```python
from build123d import *

# Parameters (mm, degrees)
SKETCH1_W           = 88.9
SKETCH1_H           = 88.9
SKETCH1_W_2         = 76.2
SKETCH1_H_2         = 76.2
BOSS_EXTRUDE1_DEPTH = 50.8
SKETCH2_W           = 88.9
SKETCH2_H           = 88.9
BOSS_EXTRUDE2_DEPTH = 6.35
SKETCH3_W           = 12.7
SKETCH3_H           = 12.7
BOSS_EXTRUDE3_DEPTH = 6.35
SKETCH4_R           = 3.175
CUT_EXTRUDE1_DEPTH  = 58.15


with BuildPart() as part:
    # Sketch1 → Boss-Extrude1 (new body)
    with BuildSketch(Plane(origin=(0, 0, 0), x_dir=(1, 0, 0), z_dir=(0, 1, 0))):
        with Locations((38.1, 38.1)):
            Rectangle(SKETCH1_W, SKETCH1_H)
        with Locations((38.1, 38.1)):
            Rectangle(SKETCH1_W_2, SKETCH1_H_2, mode=Mode.SUBTRACT)
    extrude(amount=BOSS_EXTRUDE1_DEPTH)

    # Sketch2 → Boss-Extrude2 (add)
    with BuildSketch(Plane.XZ):
        with Locations((38.1, -38.1)):
            Rectangle(SKETCH2_W, SKETCH2_H)
    extrude(amount=BOSS_EXTRUDE2_DEPTH)

    # Sketch3 → Boss-Extrude3 (add)
    with BuildSketch(Plane(origin=(0, 50.8, 0), x_dir=(1, 0, 0), z_dir=(0, 1, 0))):
        with Locations((88.9, 38.1)):
            Rectangle(SKETCH3_W, SKETCH3_H)
        with Locations((-12.7, 38.1)):
            Rectangle(SKETCH3_W, SKETCH3_H)
    extrude(amount=-BOSS_EXTRUDE3_DEPTH)

    # Sketch4 → Cut-Extrude1 (cut, through all)
    with BuildSketch(Plane(origin=(0, 50.8, 0), x_dir=(1, 0, 0), z_dir=(0, 1, 0))):
        with Locations((88.9, 38.1)):
            Circle(SKETCH4_R)
        with Locations((-12.7, 38.1)):
            Circle(SKETCH4_R)
    extrude(amount=-CUT_EXTRUDE1_DEPTH, mode=Mode.SUBTRACT)


solid = part.part
```
Source: CAD feature listing. Evaluate the final solid. Frame: model axes, mm. A direction names the side the tool comes from. Round coordinates to 2 decimals unless told otherwise and drop trailing zeros. Loops run counter-clockwise (first coordinate to the right, second up) from the corner with the lowest first, then second, coordinate; pieces in that order, holes last. Notation, with made-up numbers: M -35.5,-36.5 L -18.5,-36.5 A19 cw -18.5,-9.5 Z; hole C 43,70 d7. An arc over 180 degrees is marked long. Put each result on its own line as item: value.
(1) Section D-D, the plane y = 46.5. Return loops of the section in (x, z) (3 decimals), and give its area (3 significant figures).
Solutions:
outline: M -19.05,-44.45 L -6.35,-44.45 L -6.35,-82.55 L 82.55,-82.55 L 82.55,-44.45 L 95.25,-44.45 L 95.25,-31.75 L 82.55,-31.75 L 82.55,6.35 L -6.35,6.35 L -6.35,-31.75 L -19.05,-31.75 Z; hole C -12.7,-38.1 d6.35; hole M 0,-76.2 L 76.2,-76.2 L 76.2,0 L 0,0 Z; hole C 88.9,-38.1 d6.35
area: 2,360 mm²
(2) First-contact query: pin 1 (3 mm diameter, centred on x = -10, y = 46, fed in from +Z); pin 2 (17 mm diameter, centred on y = 17.5, z = -26, fed in from -X); pin 3 (7 mm diameter, centred on x = -15.5, y = 47, fed in from -Z); pin 4 (4 mm diameter, centred on x = 88.9, z = -38.1, fed in from -Y). Flat tips, straight axial feed; report the tip coordinate or a pass-through.
Solutions:
pin 1: z = -31.75
pin 2: x = -6.35
pin 3: z = -44.45
pin 4: through
(3) Section B-B, the plane x = 88.9. Return loops of the section in (y, z) (3 decimals), and give its area (3 significant figures).
Solutions:
outline: M 44.45,-44.45 L 50.8,-44.45 L 50.8,-41.275 L 44.45,-41.275 Z; M 44.45,-34.925 L 50.8,-34.925 L 50.8,-31.75 L 44.45,-31.75 Z
area: 40.3 mm²
(4) Access query for faces 1 (the face through (-16, 44.45, -40)), 2 (the face through (38, 25, -76.2)), 3 (the face through (86, 44.45, -40)), 4 (the face through (89, 48, -44.45)). Directions: +Z, -Z, +X, -X, +Y, -Y. A direction counts if a zero-diameter tool reaches every point of the face in a straight line with its end or side. Return the directions, or none.
Solutions:
face 1: +Z, -Z, -X, -Y
face 2: +Y
face 3: +Z, -Z, +X, -Y
face 4: -Z, +X, +Y, -Y
(5) Section A-A, the plane z = -38.1. Return loops of the section in (x, y) (3 decimals), and give its area (3 significant figures).
Solutions:
outline: M -19.05,44.45 L -15.875,44.45 L -15.875,50.8 L -19.05,50.8 Z; M -9.525,44.45 L -6.35,44.45 L -6.35,-6.35 L 82.55,-6.35 L 82.55,44.45 L 85.725,44.45 L 85.725,50.8 L 76.2,50.8 L 76.2,0 L 0,0 L 0,50.8 L -9.525,50.8 Z; M 92.075,44.45 L 95.25,44.45 L 95.25,50.8 L 92.075,50.8 Z
area: 1,290 mm²
(6) Pull-direction query (Z, two-part tool) for faces 5 (the face through (76.2, 25, -38)), 6 (the face through (37, 23, -82.55)), 7 (the face through (-0.3, 50.8, -41.6)); classes: released by +Z, released by -Z, zero draft, split by the parting line, or undercut.
Solutions:
face 5: undercut
face 6: released by -Z
face 7: zero draft
(7) Section C-C, the plane y = 30. Return loops of the section in (x, z), and give its area (3 significant figures).
Solutions:
outline: M -6.35,-82.55 L 82.55,-82.55 L 82.55,6.35 L -6.35,6.35 Z; hole M 0,-76.2 L 76.2,-76.2 L 76.2,0 L 0,0 Z
area: 2,100 mm²
(8) Ray query, line 1 (X direction, y = 48.75, z = -38.1) (3 decimals); line 2 (Z direction, x = 44.5, y = 31.5); line 3 (Z direction, x = 88.9, y = 48) (3 decimals). Return the intervals inside material, ascending. Write a range as [from, to].
Solutions:
line 1: [-19.05, -15.875], [-9.525, 0], [76.2, 85.725], [92.075, 95.25]
line 2: [-82.55, -76.2], [0, 6.35]
line 3: [-44.45, -41.275], [-34.925, -31.75]
